Autodesk Fusion 360 part; units mm, degrees
sketch "Sketch1" plane through (0, 0, 0) normal (1, 0, 0) x (0, 0, -1)
  arc A0 (30.8871, 27.0565) -> (30.1313, 27.8123) centre (14.9574, 11.8827) ccw
  arc A1 (10.989, -9.7564) -> (12.0447, -9.9237) centre (14.9574, 11.8827) ccw
  arc A2 (4.4964, -7.4711) -> (5.4488, -7.9563) centre (14.9574, 11.8827) ccw
  arc A3 (12.0447, 33.689) -> (10.989, 33.5218) centre (14.9574, 11.8827) ccw
  arc A4 (24.4289, 26.5968) -> (25.4184, 31.2364) centre (17.4515, 30.5103) ccw
  arc A5 (34.3112, 22.3437) -> (29.6716, 21.3542) centre (33.5851, 14.3767) ccw
  arc A6 (25.4184, -7.4711) -> (24.4289, -2.8315) centre (17.4515, -6.745) ccw
  arc A7 (32.4286, 10.8965) -> (32.4286, 12.8689) centre (14.9574, 11.8827) ccw
  arc A8 (36.5965, 7.9143) -> (36.7638, 8.97) centre (14.9574, 11.8827) ccw
  arc A9 (30.8871, -3.2912) -> (28.5123, 0.8155) centre (23.0856, -5.0625) ccw
  arc A10 (1.4026, 0.8155) -> (-0.9722, -3.2912) centre (6.8292, -5.0625) ccw
  arc A11 (-1.3539, 18.2195) -> (-1.9634, 16.3437) centre (14.9574, 11.8827) ccw
  arc A12 (-2.5138, 12.8689) -> (-2.5138, 10.8965) centre (14.9574, 11.8827) ccw
  arc A13 (-1.9634, 16.3437) -> (-6.6817, 15.8511) centre (-3.5292, 8.4984) ccw
  arc A14 (28.5123, 0.8155) -> (29.6716, 2.4112) centre (14.9574, 11.8827) ccw
  arc A15 (10.989, -9.7564) -> (12.0447, -9.9237) centre (14.9574, 11.8827) ccw
  arc A16 (29.6716, 2.4112) -> (34.3112, 1.4217) centre (33.5851, 9.3886) ccw
  arc A17 (8.6206, -4.4287) -> (10.4964, -5.0382) centre (14.9574, 11.8827) ccw
  arc A18 (36.7638, 8.97) -> (32.4286, 10.8965) centre (31.4935, 2.9514) ccw
  arc A19 (28.5123, 0.8155) -> (29.6716, 2.4112) centre (14.9574, 11.8827) ccw
  arc A20 (5.4859, -2.8315) -> (4.4964, -7.4711) centre (12.4634, -6.745) ccw
  arc A21 (24.4661, 31.7217) -> (21.2942, 28.194) centre (28.5615, 24.8494) ccw
  arc A22 (-0.9722, 27.0565) -> (1.4026, 22.9498) centre (6.8292, 28.8279) ccw
  arc A23 (21.2942, -4.4287) -> (24.4661, -7.9563) centre (28.5615, -1.0841) ccw
  arc A24 (25.4184, 31.2364) -> (24.4661, 31.7217) centre (14.9574, 11.8827) ccw
  arc A25 (-1.3539, 5.5459) -> (-4.8816, 2.374) centre (1.9907, -1.7214) ccw
  arc A26 (25.4184, -7.4711) -> (24.4289, -2.8315) centre (17.4515, -6.745) ccw
  arc A27 (5.4859, 26.5968) -> (3.8903, 25.4375) centre (14.9574, 11.8827) ccw
  arc A28 (-0.9722, -3.2912) -> (-0.2164, -4.047) centre (14.9574, 11.8827) ccw
  arc A29 (-6.8489, 8.97) -> (-6.6817, 7.9143) centre (14.9574, 11.8827) ccw
  arc A30 (24.4661, -7.9563) -> (25.4184, -7.4711) centre (14.9574, 11.8827) ccw
  arc A31 (10.989, 33.5218) -> (10.4964, 28.8035) centre (18.3417, 30.3693) ccw
  arc A32 (-0.2164, -4.047) -> (3.8903, -1.6722) centre (-1.9878, 3.7545) ccw
  arc A33 (18.9258, 33.5218) -> (17.8701, 33.689) centre (14.9574, 11.8827) ccw
  arc A34 (3.8903, 25.4375) -> (-0.2164, 27.8123) centre (-1.9878, 20.0109) ccw
  arc A35 (12.0447, 33.689) -> (10.989, 33.5218) centre (14.9574, 11.8827) ccw
  arc A36 (0.2433, 2.4112) -> (1.4026, 0.8155) centre (14.9574, 11.8827) ccw
  arc A37 (-0.9722, 27.0565) -> (1.4026, 22.9498) centre (6.8292, 28.8279) ccw
  arc A38 (24.4289, -2.8315) -> (26.0246, -1.6722) centre (14.9574, 11.8827) ccw
  arc A39 (-6.8489, 8.97) -> (-6.6817, 7.9143) centre (14.9574, 11.8827) ccw
  arc A40 (-4.3963, 1.4217) -> (0.2433, 2.4112) centre (-3.6702, 9.3886) ccw
  arc A41 (1.4026, 0.8155) -> (-0.9722, -3.2912) centre (6.8292, -5.0625) ccw
  arc A42 (-0.2164, 27.8123) -> (-0.9722, 27.0565) centre (14.9574, 11.8827) ccw
  arc A43 (8.6206, 28.194) -> (5.4488, 31.7217) centre (1.3533, 24.8494) ccw
  arc A44 (4.4964, 31.2364) -> (5.4859, 26.5968) centre (12.4634, 30.5103) ccw
  arc A45 (0.2433, 21.3542) -> (-4.3963, 22.3437) centre (-3.6702, 14.3767) ccw
  arc A46 (18.9258, 33.5218) -> (17.8701, 33.689) centre (14.9574, 11.8827) ccw
  arc A47 (4.4964, 31.2364) -> (5.4859, 26.5968) centre (12.4634, 30.5103) ccw
  arc A48 (19.4184, 28.8035) -> (18.9258, 33.5218) centre (11.5731, 30.3693) ccw
  arc A49 (-1.9634, 7.4217) -> (-1.3539, 5.5459) centre (14.9574, 11.8827) ccw
  arc A50 (10.4964, -5.0382) -> (10.989, -9.7564) centre (18.3417, -6.604) ccw
  arc A51 (30.8871, 27.0565) -> (30.1313, 27.8123) centre (14.9574, 11.8827) ccw
  arc A52 (-4.8816, 2.374) -> (-4.3963, 1.4217) centre (14.9574, 11.8827) ccw
  arc A53 (21.2942, 28.194) -> (19.4184, 28.8035) centre (14.9574, 11.8827) ccw
  arc A54 (-0.9722, -3.2912) -> (-0.2164, -4.047) centre (14.9574, 11.8827) ccw
  arc A55 (30.1313, 27.8123) -> (26.0246, 25.4375) centre (31.9027, 20.0109) ccw
  arc A56 (-4.3963, 22.3437) -> (-4.8816, 21.3913) centre (14.9574, 11.8827) ccw
  arc A57 (13.9712, 29.3539) -> (12.0447, 33.689) centre (6.0261, 28.4187) ccw
  arc A58 (-2.5138, 10.8965) -> (-6.8489, 8.97) centre (-1.5786, 2.9514) ccw
  arc A59 (13.9712, 29.3539) -> (12.0447, 33.689) centre (6.0261, 28.4187) ccw
  arc A60 (34.7964, 21.3913) -> (34.3112, 22.3437) centre (14.9574, 11.8827) ccw
  arc A61 (8.6206, 28.194) -> (5.4488, 31.7217) centre (1.3533, 24.8494) ccw
  arc A62 (-2.5138, 12.8689) -> (-2.5138, 10.8965) centre (14.9574, 11.8827) ccw
  arc A63 (19.4184, -5.0382) -> (21.2942, -4.4287) centre (14.9574, 11.8827) ccw
  arc A64 (13.9712, -5.5885) -> (15.9436, -5.5885) centre (14.9574, 11.8827) ccw
  arc A65 (30.1313, 27.8123) -> (26.0246, 25.4375) centre (31.9027, 20.0109) ccw
  arc A66 (19.4184, 28.8035) -> (18.9258, 33.5218) centre (11.5731, 30.3693) ccw
  arc A67 (18.9258, -9.7564) -> (19.4184, -5.0382) centre (11.5731, -6.604) ccw
  arc A68 (-6.6817, 7.9143) -> (-1.9634, 7.4217) centre (-3.5292, 15.267) ccw
  arc A69 (5.4488, 31.7217) -> (4.4964, 31.2364) centre (14.9574, 11.8827) ccw
  arc A70 (12.0447, -9.9237) -> (13.9712, -5.5885) centre (6.0261, -4.6534) ccw
  arc A71 (36.7638, 14.7954) -> (36.5965, 15.8511) centre (14.9574, 11.8827) ccw
  arc A72 (32.4286, 12.8689) -> (36.7638, 14.7954) centre (31.4935, 20.814) ccw
  arc A73 (10.4964, 28.8035) -> (8.6206, 28.194) centre (14.9574, 11.8827) ccw
  arc A74 (15.9436, -5.5885) -> (17.8701, -9.9237) centre (23.8887, -4.6534) ccw
  arc A75 (17.8701, -9.9237) -> (18.9258, -9.7564) centre (14.9574, 11.8827) ccw
  arc A76 (1.4026, 22.9498) -> (0.2433, 21.3542) centre (14.9574, 11.8827) ccw
  arc A77 (26.0246, 25.4375) -> (24.4289, 26.5968) centre (14.9574, 11.8827) ccw
  arc A78 (17.8701, 33.689) -> (15.9436, 29.3539) centre (23.8887, 28.4187) ccw
  arc A79 (32.4286, 10.8965) -> (32.4286, 12.8689) centre (14.9574, 11.8827) ccw
  arc A80 (15.9436, 29.3539) -> (13.9712, 29.3539) centre (14.9574, 11.8827) ccw
  arc A81 (24.4289, 26.5968) -> (25.4184, 31.2364) centre (17.4515, 30.5103) ccw
  arc A82 (32.4286, 12.8689) -> (36.7638, 14.7954) centre (31.4935, 20.814) ccw
  arc A83 (25.4184, 31.2364) -> (24.4661, 31.7217) centre (14.9574, 11.8827) ccw
  arc A84 (36.7638, 14.7954) -> (36.5965, 15.8511) centre (14.9574, 11.8827) ccw
  arc A85 (34.7964, 21.3913) -> (34.3112, 22.3437) centre (14.9574, 11.8827) ccw
  arc A86 (31.2688, 18.2195) -> (34.7964, 21.3913) centre (27.9242, 25.4868) ccw
  arc A87 (28.5123, 22.9498) -> (30.8871, 27.0565) centre (23.0856, 28.8279) ccw
  arc A88 (34.3112, 22.3437) -> (29.6716, 21.3542) centre (33.5851, 14.3767) ccw
  arc A89 (31.8783, 16.3437) -> (31.2688, 18.2195) centre (14.9574, 11.8827) ccw
  arc A90 (36.5965, 15.8511) -> (31.8783, 16.3437) centre (33.4441, 8.4984) ccw
  arc A91 (29.6716, 21.3542) -> (28.5123, 22.9498) centre (14.9574, 11.8827) ccw
  arc A92 (-4.8816, 21.3913) -> (-1.3539, 18.2195) centre (1.9907, 25.4868) ccw
  arc A93 (4.4964, -7.4711) -> (5.4488, -7.9563) centre (14.9574, 11.8827) ccw
  arc A94 (30.1313, -4.047) -> (30.8871, -3.2912) centre (14.9574, 11.8827) ccw
  arc A95 (5.4859, -2.8315) -> (4.4964, -7.4711) centre (12.4634, -6.745) ccw
  arc A96 (5.4488, -7.9563) -> (8.6206, -4.4287) centre (1.3533, -1.0841) ccw
  arc A97 (26.0246, -1.6722) -> (30.1313, -4.047) centre (31.9027, 3.7545) ccw
  arc A98 (-1.3539, 18.2195) -> (-1.9634, 16.3437) centre (14.9574, 11.8827) ccw
  arc A99 (10.989, 33.5218) -> (10.4964, 28.8035) centre (18.3417, 30.3693) ccw
  arc A100 (30.1313, -4.047) -> (30.8871, -3.2912) centre (14.9574, 11.8827) ccw
  arc A101 (-4.3963, 22.3437) -> (-4.8816, 21.3913) centre (14.9574, 11.8827) ccw
  arc A102 (21.2942, -4.4287) -> (24.4661, -7.9563) centre (28.5615, -1.0841) ccw
  arc A103 (15.9436, -5.5885) -> (17.8701, -9.9237) centre (23.8887, -4.6534) ccw
  arc A104 (29.6716, 2.4112) -> (34.3112, 1.4217) centre (33.5851, 9.3886) ccw
  arc A105 (18.9258, -9.7564) -> (19.4184, -5.0382) centre (11.5731, -6.604) ccw
  arc A106 (3.8903, -1.6722) -> (5.4859, -2.8315) centre (14.9574, 11.8827) ccw
  arc A107 (31.8783, 7.4217) -> (36.5965, 7.9143) centre (33.4441, 15.267) ccw
  arc A108 (34.3112, 1.4217) -> (34.7964, 2.374) centre (14.9574, 11.8827) ccw
  arc A109 (1.4026, 22.9498) -> (0.2433, 21.3542) centre (14.9574, 11.8827) ccw
  arc A110 (0.2433, 21.3542) -> (-4.3963, 22.3437) centre (-3.6702, 14.3767) ccw
  arc A111 (34.7964, 2.374) -> (31.2688, 5.5459) centre (27.9242, -1.7214) ccw
  arc A112 (24.4661, -7.9563) -> (25.4184, -7.4711) centre (14.9574, 11.8827) ccw
  arc A113 (26.0246, -1.6722) -> (30.1313, -4.047) centre (31.9027, 3.7545) ccw
  arc A114 (31.2688, 5.5459) -> (31.8783, 7.4217) centre (14.9574, 11.8827) ccw
  arc A115 (10.4964, -5.0382) -> (10.989, -9.7564) centre (18.3417, -6.604) ccw
  arc A116 (12.0447, -9.9237) -> (13.9712, -5.5885) centre (6.0261, -4.6534) ccw
  arc A117 (-6.6817, 15.8511) -> (-6.8489, 14.7954) centre (14.9574, 11.8827) ccw
  arc A118 (34.3112, 1.4217) -> (34.7964, 2.374) centre (14.9574, 11.8827) ccw
  arc A119 (24.4289, -2.8315) -> (26.0246, -1.6722) centre (14.9574, 11.8827) ccw
  arc A120 (-6.8489, 14.7954) -> (-2.5138, 12.8689) centre (-1.5786, 20.814) ccw
  arc A121 (-4.8816, 2.374) -> (-4.3963, 1.4217) centre (14.9574, 11.8827) ccw
  arc A122 (10.4964, 28.8035) -> (8.6206, 28.194) centre (14.9574, 11.8827) ccw
  arc A123 (5.4859, 26.5968) -> (3.8903, 25.4375) centre (14.9574, 11.8827) ccw
  arc A124 (36.5965, 7.9143) -> (36.7638, 8.97) centre (14.9574, 11.8827) ccw
  arc A125 (3.8903, -1.6722) -> (5.4859, -2.8315) centre (14.9574, 11.8827) ccw
  arc A126 (-2.5138, 10.8965) -> (-6.8489, 8.97) centre (-1.5786, 2.9514) ccw
  arc A127 (5.4488, 31.7217) -> (4.4964, 31.2364) centre (14.9574, 11.8827) ccw
  arc A128 (-4.3963, 1.4217) -> (0.2433, 2.4112) centre (-3.6702, 9.3886) ccw
  arc A129 (34.7964, 2.374) -> (31.2688, 5.5459) centre (27.9242, -1.7214) ccw
  arc A130 (13.9712, -5.5885) -> (15.9436, -5.5885) centre (14.9574, 11.8827) ccw
  arc A131 (-6.6817, 7.9143) -> (-1.9634, 7.4217) centre (-3.5292, 15.267) ccw
  arc A132 (31.8783, 7.4217) -> (36.5965, 7.9143) centre (33.4441, 15.267) ccw
  arc A133 (5.4488, -7.9563) -> (8.6206, -4.4287) centre (1.3533, -1.0841) ccw
  arc A134 (0.2433, 2.4112) -> (1.4026, 0.8155) centre (14.9574, 11.8827) ccw
  arc A135 (36.7638, 8.97) -> (32.4286, 10.8965) centre (31.4935, 2.9514) ccw
  arc A136 (-0.2164, -4.047) -> (3.8903, -1.6722) centre (-1.9878, 3.7545) ccw
  arc A137 (28.5123, 22.9498) -> (30.8871, 27.0565) centre (23.0856, 28.8279) ccw
  arc A138 (19.4184, -5.0382) -> (21.2942, -4.4287) centre (14.9574, 11.8827) ccw
  arc A139 (17.8701, -9.9237) -> (18.9258, -9.7564) centre (14.9574, 11.8827) ccw
  arc A140 (30.8871, -3.2912) -> (28.5123, 0.8155) centre (23.0856, -5.0625) ccw
  arc A141 (21.2942, 28.194) -> (19.4184, 28.8035) centre (14.9574, 11.8827) ccw
  arc A142 (36.5965, 15.8511) -> (31.8783, 16.3437) centre (33.4441, 8.4984) ccw
  arc A143 (-1.9634, 16.3437) -> (-6.6817, 15.8511) centre (-3.5292, 8.4984) ccw
  arc A144 (-6.8489, 14.7954) -> (-2.5138, 12.8689) centre (-1.5786, 20.814) ccw
  arc A145 (29.6716, 21.3542) -> (28.5123, 22.9498) centre (14.9574, 11.8827) ccw
  arc A146 (8.6206, -4.4287) -> (10.4964, -5.0382) centre (14.9574, 11.8827) ccw
  arc A147 (-4.8816, 21.3913) -> (-1.3539, 18.2195) centre (1.9907, 25.4868) ccw
  arc A148 (26.0246, 25.4375) -> (24.4289, 26.5968) centre (14.9574, 11.8827) ccw
  arc A149 (3.8903, 25.4375) -> (-0.2164, 27.8123) centre (-1.9878, 20.0109) ccw
  arc A150 (17.8701, 33.689) -> (15.9436, 29.3539) centre (23.8887, 28.4187) ccw
  arc A151 (-1.9634, 7.4217) -> (-1.3539, 5.5459) centre (14.9574, 11.8827) ccw
  arc A152 (15.9436, 29.3539) -> (13.9712, 29.3539) centre (14.9574, 11.8827) ccw
  arc A153 (31.8783, 16.3437) -> (31.2688, 18.2195) centre (14.9574, 11.8827) ccw
  arc A154 (-6.6817, 15.8511) -> (-6.8489, 14.7954) centre (14.9574, 11.8827) ccw
  arc A155 (-1.3539, 5.5459) -> (-4.8816, 2.374) centre (1.9907, -1.7214) ccw
  arc A156 (24.4661, 31.7217) -> (21.2942, 28.194) centre (28.5615, 24.8494) ccw
  arc A157 (-0.2164, 27.8123) -> (-0.9722, 27.0565) centre (14.9574, 11.8827) ccw
  arc A158 (31.2688, 18.2195) -> (34.7964, 21.3913) centre (27.9242, 25.4868) ccw
  arc A159 (31.2688, 5.5459) -> (31.8783, 7.4217) centre (14.9574, 11.8827) ccw
  circle A160 centre (14.9574, 11.8827) radius 2.75
  dimension "d4" = 5.5
extrude "Extrude1" add sketch "Sketch1" along normal blind 6
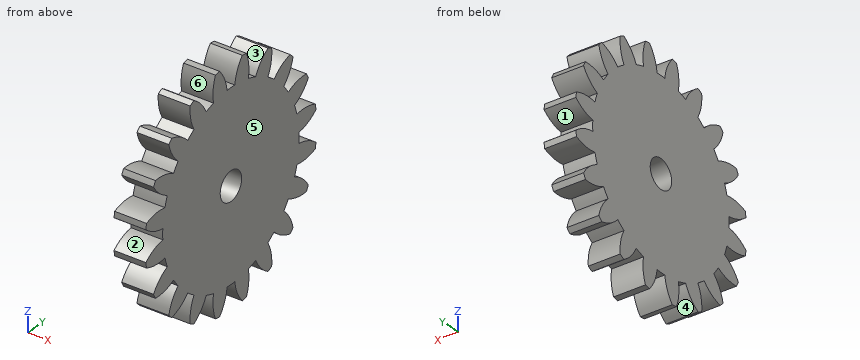
Input: part model. Units: mm. Frame: model coordinates. Face numbers are marked on the shaded views. A direction names the side the tool comes from. Give positions to 0.01 mm unless a question says otherwise; leave off trailing zeros. Order: outer loops, then holes, each group sorted by start corner. A loop starts at its lowest first (then second) coordinate and runs counter-clockwise, first axis right, second up. Notation, with made-up numbers: (81, 15) -> (115, 15) arc R18 cw to (115, 46) -> close; hole circle Ø5 at (8.5, 72.25). An arc over 180 degrees is marked (long way). Use one line per item in the form item = value.
1) Section D-D, the plane z = -7. Return loops of the section in (x, y).
Response values:
outline = (0, -6.75) -> (6, -6.75) -> (6, 30.52) -> (0, 30.52) -> close
2) Reachability of the marked faces 1, 2 and 3 from +Z, -Z, +X, -X, +Y, -Y: full face, straight path, thin tool, end or side. Return the list, or none.
Response values:
face_1 = +X, -X, +Y
face_2 = +X, -X, -Y
face_3 = +Z, +X, -X
3) Section C-C, the plane z = 3.5. Return loops of the section in (x, y), and give its area (3 significant figures).
Response values:
outline = (0, 1.39) -> (6, 1.39) -> (6, 4.1) -> (0, 4.1) -> close; (0, 7.27) -> (6, 7.27) -> (6, 10.72) -> (0, 10.72) -> close; (0, 13.05) -> (6, 13.05) -> (6, 16.5) -> (0, 16.5) -> close; (0, 19.67) -> (6, 19.67) -> (6, 22.37) -> (0, 22.37) -> close
area = 73.9 mm^2
4) Section A-A, the plane y = 30.5. Return loops of the section in (x, z), and give its area (3 significant figures).
Response values:
outline = (0, -25.45) -> (6, -25.45) -> (6, -22.9) -> (0, -22.9) -> close; (0, -19.57) -> (6, -19.57) -> (6, -16.16) -> (0, -16.16) -> close; (0, -13.75) -> (6, -13.75) -> (6, -10.34) -> (0, -10.34) -> close; (0, -7.02) -> (6, -7.02) -> (6, -4.46) -> (0, -4.46) -> close
area = 71.5 mm^2
5) Line query: probe 1 along Z at (x, y) = (3.6, 30.5); probe 2 along Z at (x, y) = (0.35, 31.5); probe 3 along Z at (x, y) = (2.45, -3). Output: solid intervals per line, ascending.
Response values:
probe_1 = -25.45 to -22.9, -19.57 to -16.16, -13.75 to -10.34, -7.02 to -4.46
probe_2 = -24.92 to -24.12, -19.49 to -16.51, -13.41 to -10.42, -5.8 to -5
probe_3 = -30.82 to -27.62, -24.52 to -5.39, -2.3 to 0.9
6) Mould query, pull axis Z, two halves, no side actions, for the marked faces 4, 5 and 6. Classes: pulls with the +Z half, pulls with the -Z half, needs draft (parallel to the pull), parting line crosses it, or undercut.
Response values:
face_4 = pulls with the -Z half
face_5 = needs draft
face_6 = undercut
7) Section B-B, the plane y = 14. Return loops of the section in (x, z).
Response values:
outline = (0, -35.69) -> (6, -35.69) -> (6, -16.71) -> (0, -16.71) -> close; (0, -13.2) -> (6, -13.2) -> (6, 5.77) -> (0, 5.77) -> close
8) First-contact query: pin 1 Ø1 at (x, z) = (5, -15) entering from +Y; pin 2 Ø3 at (x, z) = (3, -7) entering from -Y; pin 3 Ø1 at (x, y) = (4.5, -5.5) entering from +Z. Flat tips, straight axial feed; report the tip coordinate or a pass-through.
Response values:
pin_1 = 29.38
pin_2 = -7.93
pin_3 = -4.5
